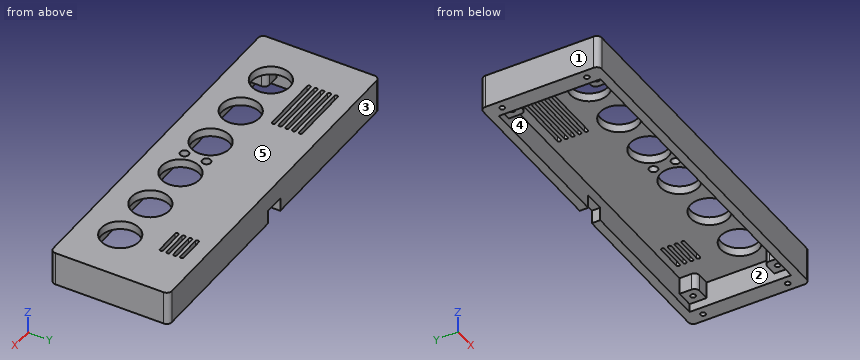
from build123d import *

# Parameters (mm, degrees)
SKETCH_1_W          = 210
SKETCH_1_H          = 70
EXTRUDE_1_DEPTH     = 20
FILLET_1_R          = 3
SKETCH_2_W          = 190
SKETCH_2_H          = 60
CUT_EXTRUDE_1_DEPTH = 15
SKETCH_3_R          = 1.5
CUT_EXTRUDE_2_DEPTH = 8
SKETCH_4_W          = 12
SKETCH_4_H          = 8
CUT_EXTRUDE_3_DEPTH = 5
SKETCH_5_R          = 11.25
SKETCH_5_R_2        = 2.5
CUT_EXTRUDE_4_DEPTH = 10
EXTRUDE_2_DEPTH     = 10
SKETCH_8_R          = 1.5
CUT_EXTRUDE_5_DEPTH = 8


with BuildPart() as part:
    # 草图1 → 凸台-拉伸1 (new body)
    with BuildSketch(Plane.XY):
        with Locations((75, 11.5)):
            Rectangle(SKETCH_1_W, SKETCH_1_H)
    extrude(amount=EXTRUDE_1_DEPTH)

    # 圆角1
    fillet_1_edges = [part.edges().sort_by_distance(p)[0] for p in [
        (-30, 46.5, 10),
        (180, 46.5, 10),
        (180, -23.5, 10),
        (-30, -23.5, 10),
    ]]
    fillet(fillet_1_edges, radius=FILLET_1_R)

    # 草图2 → 切除-拉伸1 (cut)
    with BuildSketch(Plane.XY):
        with Locations((75, 11.5)):
            Rectangle(SKETCH_2_W, SKETCH_2_H)
    extrude(amount=CUT_EXTRUDE_1_DEPTH, mode=Mode.SUBTRACT)

    # 草图3 → 切除-拉伸2 (cut)
    with BuildSketch(Plane.XY):
        with Locations((-25, 36.5)):
            Circle(SKETCH_3_R)
        with Locations((175, 36.5)):
            Circle(SKETCH_3_R)
        with Locations((-25, -13.5)):
            Circle(SKETCH_3_R)
        with Locations((175, -13.5)):
            Circle(SKETCH_3_R)
    extrude(amount=CUT_EXTRUDE_2_DEPTH, mode=Mode.SUBTRACT)

    # 草图4 → 切除-拉伸3 (cut)
    with BuildSketch(Plane(origin=(0, 46.5, 0), x_dir=(1, 0, 0), z_dir=(0, 1, 0))):
        with Locations((75, -4)):
            Rectangle(SKETCH_4_W, SKETCH_4_H)
    extrude(amount=-CUT_EXTRUDE_3_DEPTH, mode=Mode.SUBTRACT)

    # 草图5 → 切除-拉伸4 (cut)
    with BuildSketch(Plane.XY.offset(20)):
        Circle(SKETCH_5_R)
        with Locations((30, 0)):
            Circle(SKETCH_5_R)
        with Locations((60, 0)):
            Circle(SKETCH_5_R)
        with Locations((90, 0)):
            Circle(SKETCH_5_R)
        with Locations((120, 0)):
            Circle(SKETCH_5_R)
        with Locations((150, 0)):
            Circle(SKETCH_5_R)
        with Locations((75, -6.5)):
            Circle(SKETCH_5_R_2)
        with Locations((75, 6.5)):
            Circle(SKETCH_5_R_2)
        with BuildLine():
            Line((-5, 36.5), (30, 36.5))
            ThreePointArc((30, 36.5), (31, 35.5), (30, 34.5))
            Line((30, 34.5), (-5, 34.5))
            ThreePointArc((-5, 34.5), (-6, 35.5), (-5, 36.5))
        make_face()
        with BuildLine():
            Line((-5, 32.5), (30, 32.5))
            ThreePointArc((30, 32.5), (31, 31.5), (30, 30.5))
            Line((30, 30.5), (-5, 30.5))
            ThreePointArc((-5, 30.5), (-6, 31.5), (-5, 32.5))
        make_face()
        with BuildLine():
            Line((-5, 28.5), (30, 28.5))
            ThreePointArc((30, 28.5), (31, 27.5), (30, 26.5))
            Line((30, 26.5), (-5, 26.5))
            ThreePointArc((-5, 26.5), (-6, 27.5), (-5, 28.5))
        make_face()
        with BuildLine():
            Line((-5, 24.5), (30, 24.5))
            ThreePointArc((30, 24.5), (31, 23.5), (30, 22.5))
            Line((30, 22.5), (-5, 22.5))
            ThreePointArc((-5, 22.5), (-6, 23.5), (-5, 24.5))
        make_face()
        with BuildLine():
            Line((-5, 20.5), (30, 20.5))
            ThreePointArc((30, 20.5), (31, 19.5), (30, 18.5))
            Line((30, 18.5), (-5, 18.5))
            ThreePointArc((-5, 18.5), (-6, 19.5), (-5, 20.5))
        make_face()
        with BuildLine():
            Line((135, 37.5), (150, 37.5))
            ThreePointArc((150, 37.5), (151, 36.5), (150, 35.5))
            Line((150, 35.5), (135, 35.5))
            ThreePointArc((135, 35.5), (134, 36.5), (135, 37.5))
        make_face()
        with BuildLine():
            Line((135, 33.5), (150, 33.5))
            ThreePointArc((150, 33.5), (151, 32.5), (150, 31.5))
            Line((150, 31.5), (135, 31.5))
            ThreePointArc((135, 31.5), (134, 32.5), (135, 33.5))
        make_face()
        with BuildLine():
            Line((135, 29.5), (150, 29.5))
            ThreePointArc((150, 29.5), (151, 28.5), (150, 27.5))
            Line((150, 27.5), (135, 27.5))
            ThreePointArc((135, 27.5), (134, 28.5), (135, 29.5))
        make_face()
        with BuildLine():
            Line((135, 25.5), (150, 25.5))
            ThreePointArc((150, 25.5), (151, 24.5), (150, 23.5))
            Line((150, 23.5), (135, 23.5))
            ThreePointArc((135, 23.5), (134, 24.5), (135, 25.5))
        make_face()
    extrude(amount=-CUT_EXTRUDE_4_DEPTH, mode=Mode.SUBTRACT)

    # 草图6 → 凸台-拉伸2 (add)
    with BuildSketch(Plane.XY.offset(15)):
        with BuildLine():
            Line((-20, 31.5), (-13, 31.5))
            ThreePointArc((-13, 31.5), (-10.878679656, 32.378679656), (-10, 34.5))
            Line((-10, 34.5), (-10, 41.5))
            Line((-10, 41.5), (-20, 41.5))
            Line((-20, 41.5), (-20, 31.5))
        make_face()
        with BuildLine():
            Line((170, 41.5), (170, 31.5))
            Line((170, 31.5), (163, 31.5))
            ThreePointArc((163, 31.5), (160.878679656, 32.378679656), (160, 34.5))
            Line((160, 34.5), (160, 41.5))
            Line((160, 41.5), (170, 41.5))
        make_face()
        with BuildLine():
            Line((-20, -8.5), (-13, -8.5))
            ThreePointArc((-13, -8.5), (-10.878679656, -9.378679656), (-10, -11.5))
            Line((-10, -11.5), (-10, -18.5))
            Line((-10, -18.5), (-20, -18.5))
            Line((-20, -18.5), (-20, -8.5))
        make_face()
        with BuildLine():
            Line((170, -18.5), (160, -18.5))
            Line((160, -18.5), (160, -11.5))
            ThreePointArc((160, -11.5), (160.878679656, -9.378679656), (163, -8.5))
            Line((163, -8.5), (170, -8.5))
            Line((170, -8.5), (170, -18.5))
        make_face()
    extrude(amount=-EXTRUDE_2_DEPTH)

    # 草图8 → 切除-拉伸5 (cut)
    with BuildSketch(Plane(origin=(0, 0, 5), x_dir=(-1, 0, 0), z_dir=(0, 0, -1))):
        with Locations((-165, 36.5)):
            Circle(SKETCH_8_R)
        with Locations((15, 36.5)):
            Circle(SKETCH_8_R)
        with Locations((-165, -13.5)):
            Circle(SKETCH_8_R)
        with Locations((15, -13.5)):
            Circle(SKETCH_8_R)
    extrude(amount=-CUT_EXTRUDE_5_DEPTH, mode=Mode.SUBTRACT)


solid = part.part
CAD build for the part. Positions are in the model's coordinates, mm. Face numbers are marked on the shaded views. A direction names the side the tool comes from. Round coordinates to 2 decimals unless told otherwise and drop trailing zeros. Write each loop counter-clockwise with the first axis right and the second up, starting at its lowest first coordinate (ties: lowest second). Pieces come first, ordered by that corner, then holes.
(1) Slice it at B-B, the plane y = 0. Count the separate pieces of the cut face and the enclosed holes in it, and give its area (3 significant figures).
(2) Mould opens along Y. For the marked faces 1, 2 and 3 say: pulls with the +Y half, pulls with the -Y half, needs draft (parallel to the pull), parting line crosses it, or undercut.
(3) Slice it at C-C, the plane z = 3. Write the cut outline in (x, y), and give its area (3 significant figures).
(4) Drop flat-ended pins along their axis: P1, Ø2, axis at x = 92.5, y = 39, coming from the -Z side; P2, Ø8, axis at x = -15.5, y = 36, coming from the -Z side; P3, Ø0.9, axis at x = -15, y = 36.5, coming from the -Z side. Give the stop position or say it passes through.
(5) Slice it at D-D, the plane x = 118. Write the cut outline in (y, z), and give its area (3 significant figures).
(6) Probe line 1 along Y through (x, z) = (-25, 2.25); line 2 along Y through (x, z) = (-15, 8.5); line 3 along X through (y, z) = (32, 3.5). List the from-to ranges inside material, lowest first.
(7) Slice it at A-A, the plane x = 60. Write the cut outline in (y, z).
(8) 3-axis set-ups, long thin cutter, end or side, ignore diameter. For the marked faces 4 and 5: which of +Z, -Z, +X, -X, +Y, -Y reach the whole face in a straight line?
From the geometry:
1. separate pieces: 7
1. enclosed holes: 0
1. area: 675 mm2
2. face 1: needs draft
2. face 2: undercut
2. face 3: pulls with the +Y half
3. outline: (-30, -20.5) arc R3 ccw to (-27, -23.5) - (177, -23.5) arc R3 ccw to (180, -20.5) - (180, 43.5) arc R3 ccw to (177, 46.5) - (81, 46.5) - (81, 41.5) - (170, 41.5) - (170, -18.5) - (-20, -18.5) - (-20, 41.5) - (69, 41.5) - (69, 46.5) - (-27, 46.5) arc R3 ccw to (-30, 43.5) - close; hole circle Ø3 at (-25, -13.5); hole circle Ø3 at (-25, 36.5); hole circle Ø3 at (175, -13.5); hole circle Ø3 at (175, 36.5)
3. area: 3,200 mm2
4. P1: stops at z = 15
4. P2: stops at z = 5
4. P3: stops at z = 13
5. outline: (-23.5, 0) - (-18.5, 0) - (-18.5, 15) - (-11.07, 15) - (-11.07, 20) - (-23.5, 20) - close; (11.07, 15) - (41.5, 15) - (41.5, 0) - (46.5, 0) - (46.5, 20) - (11.07, 20) - close
5. area: 389 mm2
6. line 1: y = -23.5 to -15, -12 to 35, 38 to 46.5
6. line 2: y = -23.5 to -15, -12 to -8.5, 31.5 to 35, 38 to 46.5
6. line 3: x = -30 to -20, 170 to 180
7. outline: (-23.5, 0) - (-18.5, 0) - (-18.5, 15) - (-11.25, 15) - (-11.25, 20) - (-23.5, 20) - close; (11.25, 15) - (41.5, 15) - (41.5, 0) - (46.5, 0) - (46.5, 20) - (11.25, 20) - close
8. face 4: -Z
8. face 5: +Z, +X, -X, +Y, -Y
